Here's how the part is built. I have some questions about the finished solid (model axes, mm). A direction names the side the tool comes from. Round coordinates to 2 decimals unless told otherwise and drop trailing zeros. Write each loop counter-clockwise with the first axis right and the second up, starting at its lowest first coordinate (ties: lowest second). Pieces come first, ordered by that corner, then holes. Notation, with made-up numbers: M 38,-39 L 48,-39 A23 cw 48,-7 Z; hole C -36,20.25 d1. An arc over 180 degrees is marked long. Write item = value, one per line. Start each with the question number.
(1) On a 3-axis mill with a long thin cutter (end or side, diameter ignored), from which of +Z, -Z, +X, -X, +Y, -Y can I reach the whole of each face in a straight line? I mean faces 1 (the flat face through (0, -11, -21.57)), 2 (the cylindrical face through (-0.228, -10.353, -31.055)), 3 (the flat face through (2.586, -23.366, -30.841)), 4 (the flat face through (-17.367, -2.129, -23.802)). Say none if no direction works.
(2) I want a section at A-A (y = -2.75). List the corners of the cut face in (x, z) for me, and give its area (3 significant figures).
(3) I want a section at C-C (z = 0). List the corners of the cut face in (x, y) for me, and give its area (3 significant figures).
(4) I need wall thicknesses on line 1 along Z through (x, y) = (0, -6.5); line 2 along Z through (x, y) = (1, -10.5); line 3 along X through (y, z) = (-1.25, -14). Which ranges of each line are inside material? Lowest first, please.
(5) Will these pins go through, and if not, where does the flat tip stop? pin 1 Ø1 at (x, y) = (26, -23) entering from -Z; pin 2 Ø3.5 at (x, y) = (-1, -22) entering from +Z; pin 3 Ø1.7 at (x, y) = (0.5, -23) entering from -Z; pin 4 Ø3 at (x, z) = (0, -29.32) entering from +Y.
(6) If we mould it in two halves opening along Z, with no side actions, what happens to faces 5 (the flat face through (-2.61, -23.37, -30.8)), 6 (the flat face through (-24.915, -2.129, -18.48)), 7 (the flat face through (2, 0, -22))? For each: released by +Z, released by -Z, zero draft, split by the parting line, or undercut.
(7) I want a section at B-B (x = 0). List the corners of the cut face in (y, z) for me.
```python
from build123d import *

# Parameters (mm, degrees)
SKETCH2_R           = 32.5
BOSS_EXTRUDE1_DEPTH = 27
SKETCH3_R           = 29.5
CUT_EXTRUDE1_DEPTH  = 22
CHAMFER1_SIZE       = 3
BOSS_EXTRUDE2_DEPTH = 22
SKETCH6_W           = 52.5
SKETCH6_H           = 30.5
CUT_EXTRUDE3_DEPTH  = 23
CUT_EXTRUDE4_DEPTH  = 6
SKETCH12_W          = 4.2
SKETCH12_H          = 9.1
CUT_EXTRUDE5_DEPTH  = 10
SKETCH4_R           = 1.75
CUT_EXTRUDE2_DEPTH  = 28


with BuildPart() as part:
    # Sketch2 → Boss-Extrude1 (new body)
    with BuildSketch(Plane(origin=(0, 0, 0), x_dir=(1, 0, 0), z_dir=(0, 1, 0))):
        Circle(SKETCH2_R)
    extrude(amount=-BOSS_EXTRUDE1_DEPTH)

    # Sketch3 → Cut-Extrude1 (cut)
    with BuildSketch(Plane(origin=(0, 0, 0), x_dir=(1, 0, 0), z_dir=(0, 1, 0))):
        Circle(SKETCH3_R)
    extrude(amount=-CUT_EXTRUDE1_DEPTH, mode=Mode.SUBTRACT)

    # Chamfer1
    chamfer1_edges = [part.edges().sort_by_distance(p)[0] for p in [
        (-32.5, -27, 0),
    ]]
    chamfer(chamfer1_edges, length=CHAMFER1_SIZE)

    # Sketch5 → Boss-Extrude2 (add)
    with BuildSketch(Plane(origin=(0, 0, 0), x_dir=(1, 0, 0), z_dir=(0, 1, 0))):
        with BuildLine():
            Line((20.124241601, -21.57), (-20.124241601, -21.57))
            ThreePointArc((-20.124241601, -21.57), (0, -29.5), (20.124241601, -21.57))
        make_face()
    boss_extrude2 = extrude(amount=-BOSS_EXTRUDE2_DEPTH)

    # Sketch6 → Cut-Extrude3 (cut, through all)
    with BuildSketch(Plane(origin=(0, -22, 0), x_dir=(1, 0, 0), z_dir=(0, 1, 0))):
        Rectangle(SKETCH6_W, SKETCH6_H)
    extrude(amount=CUT_EXTRUDE3_DEPTH, mode=Mode.SUBTRACT)

    # Mirror1: Boss-Extrude2 across plane
    add(boss_extrude2.mirror(Plane.XY))

    # Sketch10 → Cut-Extrude4 (cut)
    with BuildSketch(Plane.XZ.offset(27)):
        Polygon((-1.732050808, -32.32), (1.732050808, -32.32), (3.464101615, -29.32), (1.732050808, -26.32), (-1.732050808, -26.32), (-3.464101615, -29.32), align=None)
        Polygon((-3.464101615, 29.32), (-1.732050808, 32.32), (1.732050808, 32.32), (3.464101615, 29.32), (1.732050808, 26.32), (-1.732050808, 26.32), align=None)
    extrude(amount=-CUT_EXTRUDE4_DEPTH, mode=Mode.SUBTRACT)

    # Sketch12 → Cut-Extrude5 (cut)
    with BuildSketch(Plane(origin=(-22.980970389, 0, -22.980970389), x_dir=(0, 1, 0), z_dir=(-0.707106781, 0, -0.707106781))):
        with Locations((-2.1, 0)):
            Rectangle(SKETCH12_W, SKETCH12_H)
    extrude(amount=-CUT_EXTRUDE5_DEPTH, mode=Mode.SUBTRACT)

    # Sketch4 → Cut-Extrude2 (cut, through all)
    with BuildSketch(Plane(origin=(0, 0, 0), x_dir=(1, 0, 0), z_dir=(0, 1, 0))):
        with Locations((0, 29.32)):
            Circle(SKETCH4_R)
        with Locations((0, -29.32)):
            Circle(SKETCH4_R)
    extrude(amount=-CUT_EXTRUDE2_DEPTH, mode=Mode.SUBTRACT)


solid = part.part
```
Returned:
q1.face_1 = +Y
q1.face_2 = +Y, -Y
q1.face_3 = -Y
q1.face_4 = -X, +Y
q2.outline = M -26.25,-15.25 L -26.25,-13.46 A29.5 cw -26.25,13.46 L -26.25,15.25 L -25.25,15.25 A29.5 cw -20.12,21.57 L 20.12,21.57 A29.5 cw 25.25,15.25 L 26.25,15.25 L 26.25,13.46 A29.5 cw 26.25,-13.46 L 26.25,-15.25 L 25.25,-15.25 A29.5 cw 20.12,-21.57 L -15.14,-21.57 L -19.54,-25.97 A32.5 ccw long -25.97,-19.54 L -23.83,-17.39 A29.5 cw -25.25,-15.25 Z; hole C 0,-29.32 d3.5; hole C 0,29.32 d3.5
q2.area = 967 mm²
q3.outline = M -32.5,-24 L -29.5,-27 L 29.5,-27 L 32.5,-24 L 32.5,0 L 29.5,0 L 29.5,-22 L -29.5,-22 L -29.5,0 L -32.5,0 Z
q3.area = 448 mm²
q4.line_1 = -32.5 to -31.07, -27.57 to -21.57, 21.57 to 27.57, 31.07 to 32.5
q4.line_2 = -32.48 to -30.76, -27.88 to -21.57, 21.57 to 27.88, 30.76 to 32.48
q4.line_3 = -29.33 to -26.25, 26.25 to 29.33
q5.pin_1 = -20.15
q5.pin_2 = 32.5
q5.pin_3 = -32.5
q5.pin_4 = through
q6.face_5 = undercut
q6.face_6 = released by -Z
q6.face_7 = zero draft
q7.outline = M -27,-26.32 L -21,-26.32 L -21,-27.57 L 0,-27.57 L 0,-21.57 L -22,-21.57 L -22,21.57 L 0,21.57 L 0,27.57 L -21,27.57 L -21,26.32 L -27,26.32 Z; M -24.18,-32.32 L -24,-32.5 L 0,-32.5 L 0,-31.07 L -21,-31.07 L -21,-32.32 Z; M -24.18,32.32 L -21,32.32 L -21,31.07 L 0,31.07 L 0,32.5 L -24,32.5 Z
